The model under review builds one solid part; all positions refer to its coordinate system, in mm. Face numbers are marked on the shaded views. A direction names the side the tool comes from. Round coordinates to 2 decimals unless told otherwise and drop trailing zeros. Write each loop counter-clockwise with the first axis right and the second up, starting at its lowest first coordinate (ties: lowest second). Pieces come first, ordered by that corner, then holes. Notation, with made-up numbers: (-32.75, 10.25) -> (10.25, 10.25) arc R22 cw to (10.25, 17.25) -> close; hole circle Ø10 at (9.25, 73.25). An arc over 180 degrees is marked (long way). Return JSON: item names as keys, results as strings. Group by question number.
1. Mouldability with a two-part tool opening along Z and no side actions: class the marked faces 1, 2 and 3 as pulls with the +Z half, pulls with the -Z half, needs draft (parallel to the pull), parting line crosses it, or undercut.
2. Tool access review of the marked faces 4 and 5: name each direction out of +Z, -Z, +X, -X, +Y, -Y from which nothing blocks a thin tool from reaching the whole face with its end or side.
3. Take a section at D-D, the plane x = 11. Write out the cut boundary in (y, z), then the cut area to 3 significant figures.
4. For line 1 along Z through (x, y) = (5.5, 44.5); line 2 along X through (y, z) = (27.5, 6.5); line 3 along X through (y, z) = (4.5, 11), list the stretches that pass through material, from the lowest coordinate up. Write a range as from..to.
5. Take a section at B-B, the plane y = 19.5. Give the number of separate pieces and of enclosed holes in the cut face, then the cut area to 3 significant figures.
6. Clearance check with flat-ended pins moving along their axes: P1, Ø2, axis at y = 27.5, z = -13, coming from the +X side; P2, Ø0.6, axis at y = 38.5, z = 14, coming from the +X side; P3, Ø1.6, axis at y = 25, z = -13, coming from the -X side; P4, Ø4, axis at x = 8.5, z = -10, coming from the +Y side. State where each tip first meets the part, or that it passes through.
7. Take a section at C-C, the plane x = 0. Write out the cut boundary in (y, z), then the cut area to 3 significant figures.
8. Take a section at A-A, the plane z = 6.25. Write out the cut boundary in (x, y).
Autodesk Inventor part; units mm, degrees
ref_plane "YZ Plane" through (0, 0, 0) normal (1, 0, 0) x (0, 1, 0)
ref_plane "XZ Plane" through (0, 0, 0) normal (0, 1, 0) x (-1, 0, 0)
ref_plane "XY Plane" through (0, 0, 0) normal (0, 0, 1) x (1, 0, 0)
sketch "Sketch1" plane through (0, 0, 0) normal (0, 1, 0) x (-1, 0, 0)
  line L0 (-25, 12.5) -> (25, 12.5)
  line L1 (25, 12.5) -> (25, -12.5)
  line L2 (25, -12.5) -> (-25, -12.5)
  line L3 (-25, -12.5) -> (-25, 12.5)
  line L4 (-25, 12.5) -> (25, -12.5) construction
  line L5 (25, 12.5) -> (-25, -12.5) construction
  line L6 (27, -14.5) -> (27, 14.5)
  line L7 (27, 14.5) -> (-27, 14.5)
  line L8 (-27, 14.5) -> (-27, -14.5)
  line L9 (-27, -14.5) -> (27, -14.5)
  point P0 (0, 0)
  dimension "d0" = 50
  dimension "d1" = 25
  dimension "d2" = 2
extrude "Extrusion1" add sketch "Sketch1" along normal blind 80
sketch "Sketch2" plane through (-27, 0, 14.5) normal (0, 0, 1) x (1, 0, 0)
  line L0 (0, 80) -> (54, 80)
  line L1 (27, 80) -> (27, 0)
  line L2 (24.5, 5) -> (24.5, 75)
  line L3 (24.5, 75) -> (29.5, 75)
  line L4 (29.5, 75) -> (29.5, 5)
  line L5 (29.5, 5) -> (24.5, 5)
  line L6 (24.5, 5) -> (29.5, 75) construction
  line L7 (24.5, 75) -> (29.5, 5) construction
  line L8 (0, 0) -> (0, 80)
  arc A0 (29.5, 72.5) -> (24.5, 72.5) centre (27, 72.5) ccw
  arc A1 (24.5, 7.5) -> (29.5, 7.5) centre (27, 7.5) ccw
  point P0 (27, 40)
  dimension "d5" = 5
  dimension "d6" = 5
extrude "Extrusion2" cut sketch "Sketch2" against normal up to surface (29 mm away) contours A0 L4 A1 L1 | L1 A1 L2 A0
sketch "Sketch3" plane through (27, 0, 14.5) normal (1, 0, 0) x (0, 0, -1)
  line L0 (0, 80) -> (29, 80)
  line L1 (14.5, 80) -> (14.5, 0)
  line L2 (27, 0) -> (2, 0)
  line L3 (17, 5) -> (17, 75)
  line L4 (17, 75) -> (12, 75)
  line L5 (12, 75) -> (12, 5)
  line L6 (12, 5) -> (17, 5)
  line L7 (17, 5) -> (12, 75) construction
  line L8 (17, 75) -> (12, 5) construction
  line L9 (0, 0) -> (0, 80)
  arc A0 (17, 72.5) -> (12, 72.5) centre (14.5, 72.5) ccw
  arc A1 (12, 7.5) -> (17, 7.5) centre (14.5, 7.5) ccw
  point P0 (14.5, 40)
  dimension "d9" = 5
  dimension "d10" = 5
extrude "Extrusion3" cut sketch "Sketch3" against normal up to surface (54 mm away) contours A0 L3 A1 L1 | L1 A1 L5 A0
fillet "Fillet1" radius 2 4 edges at (-25, 40, -12.5) (-25, 40, 12.5) (25, 40, 12.5) (25, 40, -12.5)
fillet "Fillet2" radius 3 4 edges at (27, 40, 14.5) (27, 40, -14.5) (-27, 40, -14.5) (-27, 40, 14.5)
properties part number "magazine-tower"
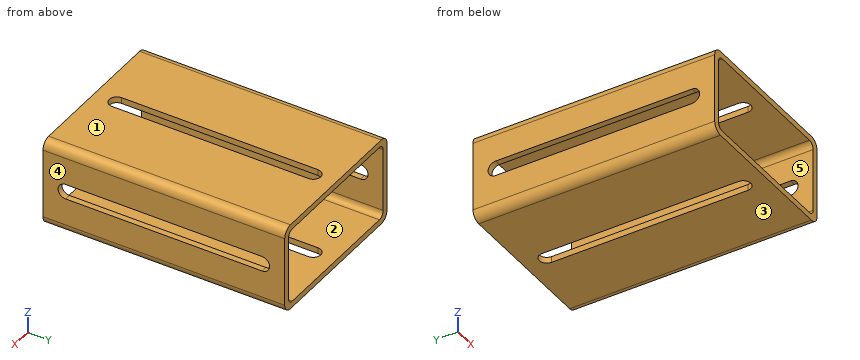
Output:
{
 "1": {"face 1": "pulls with the +Z half", "face 2": "undercut", "face 3": "pulls with the -Z half"},
 "2": {"face 4": "+Z, -Z, +X, +Y, -Y", "face 5": "+Y, -Y"},
 "3": {"outline": "(0, -14.5) -> (80, -14.5) -> (80, -12.5) -> (0, -12.5) -> close; (0, 12.5) -> (80, 12.5) -> (80, 14.5) -> (0, 14.5) -> close", "area": "320 mm^2"},
 "4": {"line 1": "z = -14.5..-12.5, 12.5..14.5", "line 2": "x = -27..-25, 25..27", "line 3": "x = -27..-24.94, 24.94..27"},
 "5": {"separate pieces": "4", "enclosed holes": "0", "area": "272 mm^2"},
 "6": {"P1": "stops at x = 26.96", "P2": "stops at x = 26.04", "P3": "stops at x = -26.92", "P4": "passes through"},
 "7": {"outline": "(0, -14.5) -> (5, -14.5) -> (5, -12.5) -> (0, -12.5) -> close; (0, 12.5) -> (5, 12.5) -> (5, 14.5) -> (0, 14.5) -> close; (75, -14.5) -> (80, -14.5) -> (80, -12.5) -> (75, -12.5) -> close; (75, 12.5) -> (80, 12.5) -> (80, 14.5) -> (75, 14.5) -> close", "area": "40.0 mm^2"},
 "8": {"outline": "(-27, 0) -> (-25, 0) -> (-25, 80) -> (-27, 80) -> close; (25, 0) -> (27, 0) -> (27, 80) -> (25, 80) -> close"}
}
